For this review, use the dimensioned drawing (mm, ordinates from the lowest corner) and the shaded views. A direction names the side the tool comes from. Give positions to 0.01 mm unless a question says otherwise; leave off trailing zeros. Loops run counter-clockwise (first coordinate to the right, second up) from the corner with the lowest first, then second, coordinate; pieces in that order, holes last. Notation, with made-up numbers: M 9,10.5 L 64,10.5 A23 cw 64,39.5 Z; hole C 15,-4 d6. An arc over 180 degrees is marked long. Use CSV: the item, a comma, the result in double quotes.
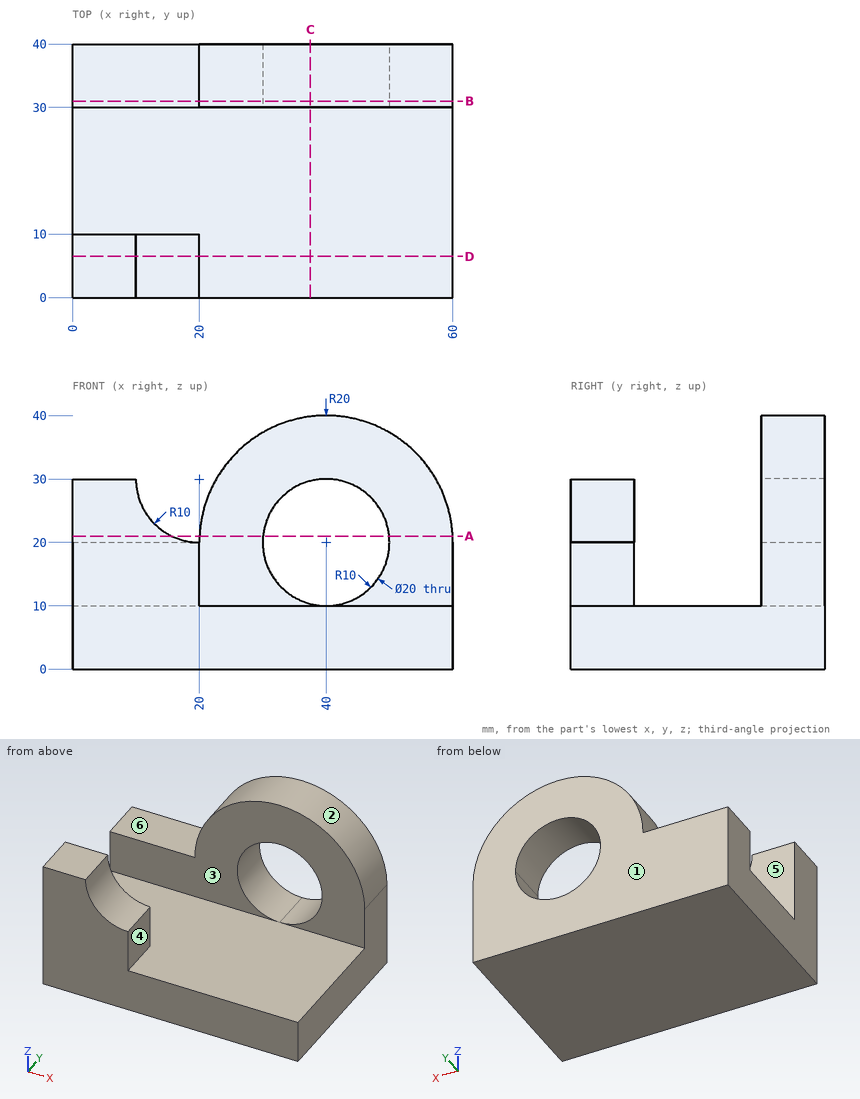
(1) The part is to be moulded in two halves that separate along Y. For the marked faces 1, 2 and 3, say which applies: released by +Y, released by -Y, zero draft, split by the parting line, or undercut.
A:
face 1,"released by +Y"
face 2,"zero draft"
face 3,"undercut"
(2) We need section B-B on y = 31. State the section outline as (x, z) points, then the cut area to 3 significant figures.
A:
outline,"M 0,0 L 60,0 L 60,20 A20 ccw 20,20 L 0,20 Z; hole C 40,20 d20"
area,"1,510 mm²"
(3) We need section D-D on y = 6.5. State the section outline as (x, z) points, then the cut area to 3 significant figures.
A:
outline,"M 0,0 L 60,0 L 60,10 L 20,10 L 20,20 A10 cw 10,30 L 0,30 Z"
area,"921 mm²"
(4) We need section C-C on x = 37.5. State the section outline as (y, z) points.
A:
outline,"M 0,0 L 40,0 L 40,10.32 L 30,10.32 L 30,10 L 0,10 Z; M 30,29.68 L 40,29.68 L 40,39.84 L 30,39.84 Z"
(5) Wall thickness on line 1 along Z through (x, y) = (40, 32.75); line 2 along Z through (x, y) = (42.5, 9.5); line 3 along Z through (x, y) = (18.5, 33): over which ranges is each line inside the solid? List them lowest first. Write a range as [from, to].
A:
line 1,"[0, 10], [30, 40]"
line 2,"[0, 10]"
line 3,"[0, 20]"
(6) We need section A-A on z = 21. State the section outline as (x, y) points, then the cut area to 3 significant figures.
A:
outline,"M 0,0 L 15.64,0 L 15.64,10 L 0,10 Z; M 20.03,30 L 30.05,30 L 30.05,40 L 20.03,40 Z; M 49.95,30 L 59.97,30 L 59.97,40 L 49.95,40 Z"
area,"357 mm²"
(7) Clearance check with flat-ended pins moving along their axes: P1, Ø8, axis at x = 3.5, y = 3, coming from the +Z side; P2, Ø3, axis at y = 6, z = 16, coming from the +X side; P3, Ø6, axis at x = 16.5, y = 20, coming from the +Z side. State where each tip first meets the part, or that it passes through.
A:
P1,"z = 30"
P2,"x = 20"
P3,"z = 10"
(8) Machinability: for the marked faces 4, 5 and 6, which of the approach directions +Z, -Z, +X, -X, +Y, -Y give a long, thin tool a straight path to every point of the face, cutting with its end or side? Answer none if there is none.
A:
face 4,"+Z, +X, -Y"
face 5,"+Z, +X, -X"
face 6,"+Z, -X, +Y"
